from build123d import *

# Parameters (mm, degrees)
SKETCH1_W           = 14
SKETCH1_H           = 4
SKETCH1_R           = 1.05
BOSS_EXTRUDE1_DEPTH = 2
SKETCH2_W           = 2
SKETCH2_H           = 4
BOSS_EXTRUDE2_DEPTH = 25.3
SKETCH3_W           = 4
SKETCH3_H           = 4
SKETCH3_R           = 1.05
BOSS_EXTRUDE3_DEPTH = 2


with BuildPart() as part:
    # Sketch1 → Boss-Extrude1 (new body)
    with BuildSketch(Plane(origin=(0, 0, 0), x_dir=(1, 0, 0), z_dir=(0, 1, 0))):
        with Locations((5, 0)):
            Rectangle(SKETCH1_W, SKETCH1_H)
        with Locations(Location((0, 0, 0), (0, 0, 270))):
            Circle(SKETCH1_R, mode=Mode.SUBTRACT)
    extrude(amount=BOSS_EXTRUDE1_DEPTH)

    # Sketch2 → Boss-Extrude2 (add)
    with BuildSketch(Plane(origin=(0, 0, 0), x_dir=(1, 0, 0), z_dir=(0, 1, 0))):
        with Locations((13, 0)):
            Rectangle(SKETCH2_W, SKETCH2_H)
    extrude(amount=BOSS_EXTRUDE2_DEPTH)

    # Sketch3 → Boss-Extrude3 (add)
    with BuildSketch(Plane(origin=(0, 25.3, 0), x_dir=(1, 0, 0), z_dir=(0, 1, 0))):
        with Locations((16, 0)):
            Rectangle(SKETCH3_W, SKETCH3_H)
        with Locations(Location((16, 0, 0), (0, 0, 270))):
            Circle(SKETCH3_R, mode=Mode.SUBTRACT)
    extrude(amount=-BOSS_EXTRUDE3_DEPTH)


solid = part.part
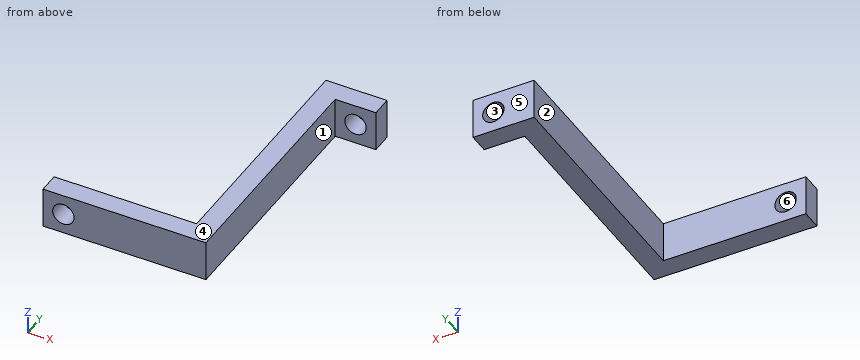
Could you check a few things on this model? Use its own coordinates, in mm. Face numbers are marked on the shaded views. A direction names the side the tool comes from. Give positions to 0.01 mm unless a question says otherwise; leave off trailing zeros. Loops run counter-clockwise (first coordinate to the right, second up) from the corner with the lowest first, then second, coordinate; pieces in that order, holes last. Notation, with made-up numbers: (31.5, 44) -> (40.5, 44) arc R9 cw to (40.5, 55) -> close; hole circle Ø7 at (11.5, 55). An arc over 180 degrees is marked (long way). Return JSON: item names as keys, results as strings.
Item 1: If we section it at C-C on z = -1.6: List the corners of the cut face in (x, y) for me, plus the area to 3 significant figures.
Geometry results:
{"outline": "(-2, 0) -> (14, 0) -> (14, 23.3) -> (18, 23.3) -> (18, 25.3) -> (12, 25.3) -> (12, 2) -> (-2, 2) -> close", "area": "86.6 mm²"}
Item 2: I need wall thicknesses on L1, parallel to X at y = 24.65, z = 0; L2, parallel to X at y = 0.5, z = 0; L3, parallel to Y at x = 15, z = 1.75. Which ranges of each line are inside material? Lowest first, please. Write a range as from..to.
Geometry results:
{"L1": "x = 12..14.95, 17.05..18", "L2": "x = -2..-1.05, 1.05..14", "L3": "y = 23.3..25.3"}
Item 3: If we section it at B-B on x = 0: List the corners of the cut face in (y, z) for me.
Geometry results:
{"outline": "(0, -2) -> (2, -2) -> (2, -1.05) -> (0, -1.05) -> close; (0, 1.05) -> (2, 1.05) -> (2, 2) -> (0, 2) -> close"}
Item 4: We'd pull the mould along Z, two halves only. Please class the marked faces 4, 5 and 6: +Z half, -Z half, draft (parallel to the pull), parting line (faces both ways), or undercut.
Geometry results:
{"face 4": "+Z half", "face 5": "draft", "face 6": "undercut"}
Item 5: If we section it at A-A on z = 0: List the corners of the cut face in (x, y) for me, plus the area to 3 significant figures.
Geometry results:
{"outline": "(-2, 0) -> (-1.05, 0) -> (-1.05, 2) -> (-2, 2) -> close; (1.05, 0) -> (14, 0) -> (14, 23.3) -> (14.95, 23.3) -> (14.95, 25.3) -> (12, 25.3) -> (12, 2) -> (1.05, 2) -> close; (17.05, 23.3) -> (18, 23.3) -> (18, 25.3) -> (17.05, 25.3) -> close", "area": "78.2 mm²"}
Item 6: Which directions (+Z, -Z, +X, -X, +Y, -Y) give clear straight access to the entire face, cutting with the end or side of a thin tool? Please do the marked faces 1, 2 and 3.
Geometry results:
{"face 1": "+Z, -Z, +X, -Y", "face 2": "+Z, -Z, -X, +Y", "face 3": "+Y, -Y"}
Item 7: I'm going to push flat-ended pins straight in: pin 1 (1.3 mm diameter, centred on x = 0, z = 0, fed in from -Y); pin 2 (2 mm diameter, centred on y = 15.5, z = 1, fed in from +X); pin 3 (2 mm diameter, centred on x = 16.5, z = 0.5, fed in from -Y). Where does each tip first touch, or does it pass through?
Geometry results:
{"pin 1": "passes through", "pin 2": "stops at x = 14", "pin 3": "stops at y = 23.3"}
Item 8: If we section it at D-D on y = 5: List the corners of the cut face in (x, z) for me.
Geometry results:
{"outline": "(12, -2) -> (14, -2) -> (14, 2) -> (12, 2) -> close"}
